Build history of the part. All positions in model axes, mm. A direction names the side the tool comes from. Round coordinates to 2 decimals unless told otherwise and drop trailing zeros. Order: outer loops, then holes, each group sorted by start corner. A loop starts at its lowest first (then second) coordinate and runs counter-clockwise, first axis right, second up. Notation, with made-up numbers: (15, 16.5) -> (19, 16.5) arc R19 ccw to (19, 43.5) -> close; hole circle Ø8 at (17.25, 65.25). An arc over 180 degrees is marked (long way). Use a Markdown table: item, result. Add a question column.
Item 1: Slice it at C-C, the plane z = 73. Give the cut face in (x, y).
Item 2: Pin check, flat tips, straight feed: pin 1 (5 mm diameter, centred on x = -7.5, y = 28.5, fed in from -Z); pin 2 (3 mm diameter, centred on y = 3.5, z = -50.5, fed in from +X); pin 3 (5.5 mm diameter, centred on x = 0, z = 0, fed in from +Y); pin 4 (20.5 mm diameter, centred on x = 0, z = -63.5, fed in from +Y). Stop position of each tip, or through.
Item 3: Probe L1, parallel to X at y = 3, z = 63; L2, parallel to X at y = 40.5, z = 0 (3 decimals); L3, parallel to Z at x = 0, y = 4.5. List the from-to ranges inside material, lowest first.
Item 4: Slice it at A-A, the plane z = 0. Give the cut face in (x, y) (3 decimals).
Item 5: Two-plate mould, pull along Z, no slides. Class faces 4 (the face through (-0.559, 3.131, -88.894)), 5 (the face through (0, 0, -54)), 6 (the face through (1.38, 3.13, -57.3)): released by +Z, released by -Z, zero draft, split by the parting line, or undercut.
Item 6: 3-axis set-ups, long thin cutter, end or side, ignore diameter. For faces 1 (the face through (6, 6.35, -66.1)), 2 (the face through (6, 6.35, 67)), 3 (the face through (-7.5, 31.742, 0.698)): which of +Z, -Z, +X, -X, +Y, -Y reach the whole face in a straight line?
Item 7: Slice it at B-B, the plane y = 13. Give the cut face in (x, z).
Autodesk Inventor part; units mm, degrees
ref_plane "YZ Plane" through (0, 0, 0) normal (1, 0, 0) x (0, 1, 0)
ref_plane "XZ Plane" through (0, 0, 0) normal (0, 1, 0) x (-1, 0, 0)
ref_plane "XY Plane" through (0, 0, 0) normal (0, 0, 1) x (1, 0, 0)
sketch "Sketch1" plane through (0, 0, 0) normal (0, 1, 0) x (-1, 0, 0)
  line L0 (0, 88.9) -> (0, -88.9) construction
  line L1 (25.4, 63.5) -> (25.4, -63.5)
  line L2 (-25.4, -63.5) -> (-25.4, 63.5)
  arc A0 (25.4, 63.5) -> (-25.4, 63.5) centre (0, 63.5) ccw
  arc A1 (-25.4, -63.5) -> (25.4, -63.5) centre (0, -63.5) ccw
  circle A2 centre (0, 63.5) radius 6.35
  circle A3 centre (0, -63.5) radius 6.35
  point P0 (0, 0)
  point P1 (0, 0)
  dimension "d0" = 127
  dimension "d1" = 12.7
  dimension "d2" = 12.7
  dimension "d3" = 25.4
extrude "BASE" add sketch "Sketch1" along normal blind 6.35
sketch "Sketch2" plane through (0, 0, 0) normal (1, 0, 0) x (0, 1, 0)
  arc A0 (0, -44.45) -> (0, 44.45) centre (0, 0) ccw
  arc A1 (0, -31.75) -> (0, 31.75) centre (0, 0) ccw
  line L0 (0, -63.5) -> (0, 63.5)
  dimension "d7" = 44.45
  dimension "d8" = 31.75
extrude "REMOVED CENTER OF BASE" cut sketch "Sketch2" along normal through all both and the other way through all contours L0 A1
extrude "ARCH" add sketch "Sketch2" along normal mid plane 63.5 contours L0 A1 A0
sketch "Sketch3" plane through (0, 0, 0) normal (0, 1, 0) x (-1, 0, 0)
  circle A0 centre (0, 0) radius 3.175
  dimension "d13" = 6.35
extrude "TOPHOLE" cut sketch "Sketch3" along normal through all
equation "\"d2\" = d1"
properties part number "ANS8-TUT-BK" material "Water"
Check sheet entries:
| question | item | result |
|---|---|---|
| 1 | outline | (-23.56, 0) -> (23.56, 0) -> (23.56, 6.35) -> (-23.56, 6.35) -> close |
| 2 | pin 1 | z = -36.05 |
| 2 | pin 2 | x = 25.4 |
| 2 | pin 3 | through |
| 2 | pin 4 | y = 6.35 |
| 3 | L1 | -25.4 to -6.33, 6.33 to 25.4 |
| 3 | L2 | -31.75 to -3.175, 3.175 to 31.75 |
| 3 | L3 | -88.9 to -69.85, -57.15 to -31.43, 31.43 to 57.15, 69.85 to 88.9 |
| 4 | outline | (-31.75, 31.75) -> (-3.175, 31.75) -> (-3.175, 44.45) -> (-31.75, 44.45) -> close; (3.175, 31.75) -> (31.75, 31.75) -> (31.75, 44.45) -> (3.175, 44.45) -> close |
| 5 | face 4 | released by -Z |
| 5 | face 5 | zero draft |
| 5 | face 6 | undercut |
| 6 | face 1 | -Z, +X, -X, +Y |
| 6 | face 2 | +Z, +X, -X, +Y |
| 6 | face 3 | +X, -X, -Y |
| 7 | outline | (-31.75, -42.51) -> (31.75, -42.51) -> (31.75, -28.97) -> (-31.75, -28.97) -> close; (-31.75, 28.97) -> (31.75, 28.97) -> (31.75, 42.51) -> (-31.75, 42.51) -> close |
